The listing builds one solid part. Answer for the finished solid, in the listing's coordinates (mm). Give positions to 0.01 mm unless a question says otherwise; leave off trailing zeros. Order: outer loops, then holes, each group sorted by start corner. A loop starts at its lowest first (then second) coordinate and runs counter-clockwise, first axis right, second up. Notation, with made-up numbers: (-7.75, 66.5) - (4.25, 66.5) arc R21 ccw to (4.25, 95.5) - close; hole circle Ø10 at (40, -12.5). An arc over 180 degrees is marked (long way). Use a Markdown table: item, result. Add a question column.
1) The mould has two halves that part along Y. Classify faces 1 (the face through (-10.2, 7.43, 43.83)), 2 (the face through (1.3, 16.2, 30.8)), 3 (the face through (618, 8, 0)), 4 (the face through (600, 26.487, 44)): released by +Y, released by -Y, zero draft, split by the parting line, or undercut.
2) Straight lines are drawn through the part: line 1 (X direction, y = 1, z = 34); line 2 (X direction, y = 18.5, z = 62.5). For each, find the intervals that lie inside material, in ascending order.
3) Find section B-B, the plane y = 17. State how many separate pieces and enclosed holes the cut face has, plus the area to 3 significant figures.
4) Flat-ended cylindrical pins translate along their axes: pin 1 (1 mm diameter, centred on y = 18, z = 17, fed in from +X); pin 2 (4 mm diameter, centred on y = 0, z = 37.5, fed in from +X). Find the tip coordinate at first contact, or state that the pin passes through.
5) Find section A-A, the plane z = 78. Determine the outline of the cut face in (x, y).
from build123d import *

# Parameters (mm, degrees)
BOSS_EXTRUDE1_DEPTH = 88.9
SKETCH2_R           = 2.5796875
CUT_EXTRUDE1_DEPTH  = 903.74963352
SKETCH3_R           = 2.5796875
CUT_EXTRUDE2_DEPTH  = 903.74963352


with BuildPart() as part:
    # Sketch1 → Boss-Extrude1 (new body)
    with BuildSketch(Plane.XY):
        Polygon((-29.256301488, 26.487163625), (1247.424473663, 26.487163625), (1209.831898512, -11.105411527), (8.336273663, -11.105411527), align=None)
    extrude(amount=BOSS_EXTRUDE1_DEPTH)

    # Sketch2 → Cut-Extrude1 (cut, through all)
    with BuildSketch(Plane(origin=(-1.384568932, -1.384568932, 0), x_dir=(0, 0, 1), z_dir=(-0.707106781, -0.707106781, 0))):
        with Locations((29.633333333, 12.834617376)):
            Circle(SKETCH2_R)
        with Locations((59.266666667, 12.834617376)):
            Circle(SKETCH2_R)
    extrude(amount=-CUT_EXTRUDE1_DEPTH, mode=Mode.SUBTRACT)

    # Sketch3 → Cut-Extrude2 (cut, through all)
    with BuildSketch(Plane(origin=(610.468655019, -610.468655019, 0), x_dir=(0, 0, -1), z_dir=(0.707106781, -0.707106781, 0))):
        with Locations((-59.266666667, 874.209592547)):
            Circle(SKETCH3_R)
        with Locations((-29.633333333, 874.209592547)):
            Circle(SKETCH3_R)
    extrude(amount=-CUT_EXTRUDE2_DEPTH, mode=Mode.SUBTRACT)


solid = part.part
The answers:
| question | item | result |
|---|---|---|
| 1 | face 1 | released by -Y |
| 1 | face 2 | undercut |
| 1 | face 3 | zero draft |
| 1 | face 4 | released by +Y |
| 2 | line 1 | -3.77 to 1221.94 |
| 2 | line 2 | -21.27 to 1239.44 |
| 3 | separate pieces | 1 |
| 3 | enclosed holes | 4 |
| 3 | area | 112,000 mm2 |
| 4 | pin 1 | x = 1239.44 |
| 4 | pin 2 | x = 1222.94 |
| 5 | outline | (-29.26, 26.49) - (8.34, -11.11) - (1209.83, -11.11) - (1247.42, 26.49) - close |
